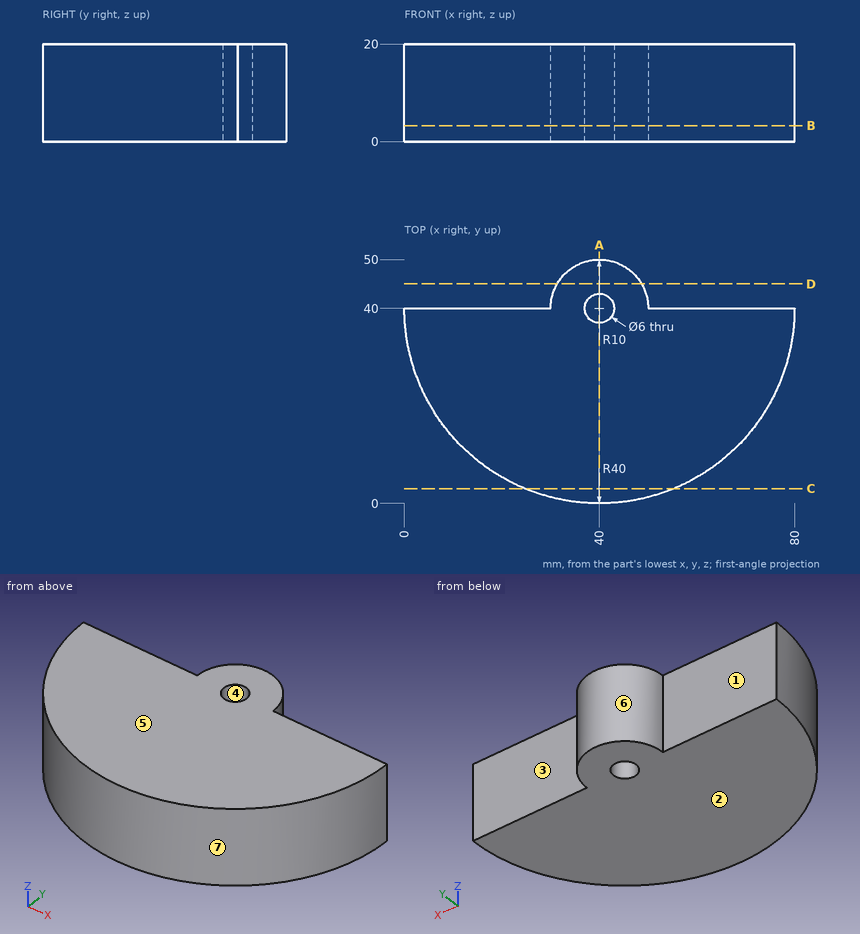
Can you work these out from the drawing? Everything is in mm from the part's minimum corner. A direction names the side the tool comes from. Give positions to 0.01 mm unless a question says otherwise; leave off trailing zeros. Order: outer loops, then holes, each group sorted by start corner. A loop starts at its lowest first (then second) coordinate and runs counter-clockwise, first axis right, second up.
1. Suppose I cut it at D-D (y = 45). List the corners of the cut face in (x, z) for me.
2. Suppose I cut it at C-C (y = 3). List the corners of the cut face in (x, z) for me, plus the area to 3 significant figures.
3. For the marked faces 1, 2 and 3, which set-ups out of +Z, -Z, +X, -X, +Y, -Y let a thin tool reach every point of the face, with its end or its side?
4. We'd pull the mould along Y, two halves only. Please class the marked faces 4, 5, 6 and 7: pulls with the +Y half, pulls with the -Y half, needs draft (parallel to the pull), parting line crosses it, or undercut.
5. Suppose I cut it at A-A (x = 40). List the corners of the cut face in (y, z) for me, plus the area to 3 significant figures.
6. Will these pins go through, and if not, where does the flat tip stop? P1, Ø12, axis at y = 33, z = 11.5, coming from the +X side; P2, Ø1.5, axis at x = 57, z = 12.5, coming from the -Y side; P3, Ø10, axis at x = 64, z = 14, coming from the +Y side; P4, Ø3.5, axis at x = 40, y = 40, coming from the +Z side.
7. Suppose I cut it at B-B (z = 3.25). List the corners of the cut face in (x, y) for me, plus the area to 3 significant figures.
8. I need wall thicknesses on L1, parallel to Y at x = 40, z = 6; L2, parallel to X at y = 7, z = 5.5; L3, parallel to X at y = 22, z = 12.5. Which ranges of each line are inside material? Lowest first, please.
Solved:
1. outline: (31.34, 0) - (48.66, 0) - (48.66, 20) - (31.34, 20) - close
2. outline: (24.8, 0) - (55.2, 0) - (55.2, 20) - (24.8, 20) - close
2. area: 608 mm2
3. face 1: +Z, -Z, -X, +Y
3. face 2: -Z, +X, -X, +Y, -Y
3. face 3: +Z, -Z, +X, +Y
4. face 4: undercut
4. face 5: needs draft
4. face 6: pulls with the +Y half
4. face 7: pulls with the -Y half
5. outline: (0, 0) - (37, 0) - (37, 20) - (0, 20) - close; (43, 0) - (50, 0) - (50, 20) - (43, 20) - close
5. area: 880 mm2
6. P1: stops at x = 79.99
6. P2: stops at y = 3.45
6. P3: stops at y = 40
6. P4: passes through
7. outline: (0, 40) arc R40 ccw to (80, 40) - (50, 40) arc R10 ccw to (30, 40) - close; hole circle Ø6 at (40, 40)
7. area: 2,640 mm2
8. L1: y = 0 to 37, 43 to 50
8. L2: x = 17.39 to 62.61
8. L3: x = 4.28 to 75.72
